from build123d import *

# Parameters (mm, degrees)
ESQUISSE1_W        = 170
ESQUISSE1_H        = 17
ESQUISSE1_R        = 2
BOSS_EXTRU_1_DEPTH = 5
CONG_1_R           = 5


with BuildPart() as part:
    # Esquisse1 → Boss.-Extru.1 (new body)
    with BuildSketch(Plane.XY):
        with Locations((85, 8.5)):
            Rectangle(ESQUISSE1_W, ESQUISSE1_H)
        with Locations((5, 5)):
            Circle(ESQUISSE1_R, mode=Mode.SUBTRACT)
        with Locations((45, 5)):
            Circle(ESQUISSE1_R, mode=Mode.SUBTRACT)
        with Locations((85, 5)):
            Circle(ESQUISSE1_R, mode=Mode.SUBTRACT)
        with Locations((125, 5)):
            Circle(ESQUISSE1_R, mode=Mode.SUBTRACT)
        with Locations((165, 5)):
            Circle(ESQUISSE1_R, mode=Mode.SUBTRACT)
    extrude(amount=BOSS_EXTRU_1_DEPTH)

    # Congé1
    cong_1_edges = [part.edges().sort_by_distance(p)[0] for p in [
        (0, 17, 2.5),
        (170, 17, 2.5),
        (170, 0, 2.5),
        (0, 0, 2.5),
    ]]
    fillet(cong_1_edges, radius=CONG_1_R)


solid = part.part
Part model, mm, in its own coordinate system. Coordinates: 2 decimals unless noted, no trailing zeros. Loops run counter-clockwise (first coordinate to the right, second up) from the corner with the lowest first, then second, coordinate; pieces in that order, holes last. Notation, with made-up numbers: M 82,-38.75 L 112,-38.75 A21 cw 112,-12.75 Z; hole C -4,48 d4. An arc over 180 degrees is marked long. Use a Markdown table: item, result. Add a question column.
Q1. Cut at A-A (x = 125). Write the cut outline in (y, z).
Q2. Mould opens along X. For faces 1 (the cylindrical face through (168, 16, 3)), 2 (the cylindrical face through (123, 5, 2)), 3 (the cylindrical face through (163, 5, 2)), 4 (the flat face through (84, 0, 2)) say: +X half, -X half, draft (parallel to the pull), parting line (faces both ways), or undercut.
Q3. Cut at B-B (z = 2.7). Write the cut outline in (x, y), and give its area (3 significant figures).
Q4. Probe L1, parallel to Y at x = 125, z = 3. List the from-to ranges inside material, lowest first.
Worked out:
| question | item | result |
|---|---|---|
| 1 | outline | M 0,0 L 3,0 L 3,5 L 0,5 Z; M 7,0 L 17,0 L 17,5 L 7,5 Z |
| 2 | face 1 | +X half |
| 2 | face 2 | undercut |
| 2 | face 3 | undercut |
| 2 | face 4 | draft |
| 3 | outline | M 0,5 A5 ccw 5,0 L 165,0 A5 ccw 170,5 L 170,12 A5 ccw 165,17 L 5,17 A5 ccw 0,12 Z; hole C 5,5 d4; hole C 45,5 d4; hole C 85,5 d4; hole C 125,5 d4; hole C 165,5 d4 |
| 3 | area | 2,810 mm2 |
| 4 | L1 | y = 0 to 3, 7 to 17 |
